Geometry check sheet. Reference: the model listing, model coordinates, mm. Round coordinates to 2 decimals unless told otherwise and drop trailing zeros. Loops run counter-clockwise (first coordinate to the right, second up) from the corner with the lowest first, then second, coordinate; pieces in that order, holes last. Notation, with made-up numbers: M 71,58.25 L 104,58.25 A18 ccw 104,84.25 Z; hole C 34,3 d11. An arc over 180 degrees is marked long. Write item = value, one per line.
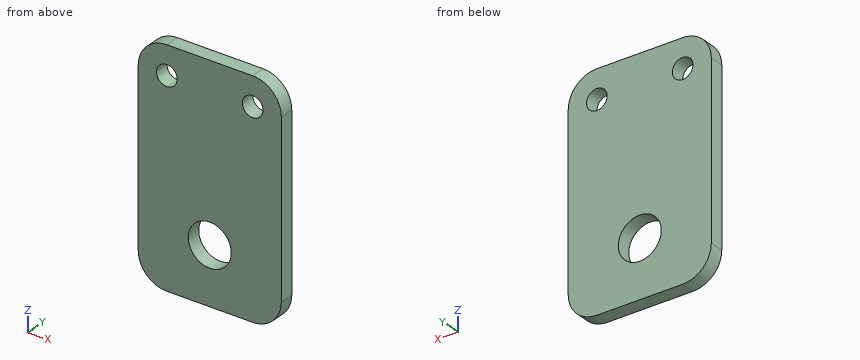
from build123d import *

# Parameters (mm, degrees)
SKETCH1_W           = 31.75
SKETCH1_H           = 50.8
SKETCH1_R           = 4.7625
SKETCH1_R_2         = 2.286
BOSS_EXTRUDE1_DEPTH = 3.175
FILLET1_R           = 6.35


with BuildPart() as part:
    # Sketch1 → Boss-Extrude1 (new body)
    with BuildSketch(Plane(origin=(0, 0, 0), x_dir=(1, 0, 0), z_dir=(0, 1, 0))):
        with Locations((15.875, 25.4)):
            Rectangle(SKETCH1_W, SKETCH1_H)
        with Locations((15.875, 38.1)):
            Circle(SKETCH1_R, mode=Mode.SUBTRACT)
        with Locations((6.35, 6.35)):
            Circle(SKETCH1_R_2, mode=Mode.SUBTRACT)
        with Locations((25.4, 6.35)):
            Circle(SKETCH1_R_2, mode=Mode.SUBTRACT)
    extrude(amount=BOSS_EXTRUDE1_DEPTH)

    # Fillet1
    fillet1_edges = [part.edges().sort_by_distance(p)[0] for p in [
        (0, 1.5875, -50.8),
        (31.75, 1.5875, -50.8),
        (31.75, 1.5875, 0),
        (0, 1.5875, 0),
    ]]
    fillet(fillet1_edges, radius=FILLET1_R)


solid = part.part
(1) Sectioned sample at D-D on x = 3. Record the cut outline in (y, z) (3 decimals), then the cut area to 3 significant figures.
Result set:
outline = M 0,-49.844 L 3.175,-49.844 L 3.175,-0.956 L 0,-0.956 Z
area = 155 mm2
(2) Sectioned sample at B-B on y = 0.85. State how many separate pieces and enclosed holes the cut face has, then the cut area to 3 significant figures.
Result set:
separate_pieces = 1
enclosed_holes = 3
area = 1,470 mm2
(3) Sectioned sample at C-C on x = 24. Record the cut outline in (y, z) (3 decimals), then the cut area to 3 significant figures.
Result set:
outline = M 0,-50.8 L 3.175,-50.8 L 3.175,-8.157 L 0,-8.157 Z; M 0,-4.543 L 3.175,-4.543 L 3.175,0 L 0,0 Z
area = 150 mm2
(4) Material ranges on line 1 along X through (y, z) = (0.55, -8); line 2 along Z through (x, y) = (20, 1.1); line 3 along Z through (x, y) = (6.5, 2.1), recorded low to high. Write a range as from..to.
Result set:
line_1 = 0..4.77, 7.93..23.82, 26.98..31.75
line_2 = -50.8..-40.48, -35.72..0
line_3 = -50.8..-8.63, -4.07..0
(5) Depth check by flat-ended pin: pin 1 Ø1.5 at (x, y) = (27.5, 2.5) entering from +Z; pin 2 Ø1.5 at (x, y) = (28.5, 2.5) entering from +Z. Enter the tip coordinate at first touch or a pass-through.
Result set:
pin_1 = -0.15
pin_2 = -0.45
